Here's how the part is built. I have some questions about the finished solid (model axes, mm). A direction names the side the tool comes from. Coordinates: 2 decimals unless noted, no trailing zeros. Order: outer loops, then holes, each group sorted by start corner. A loop starts at its lowest first (then second) coordinate and runs counter-clockwise, first axis right, second up. Notation, with made-up numbers: (3.5, 5.25) - (31.5, 5.25) arc R25 ccw to (31.5, 17.25) - close; hole circle Ø3 at (-2.75, -19.75). An arc over 180 degrees is marked (long way). Answer as CSV lines item,"result". Start each with the question number.
Item 1: I need wall thicknesses on line 1 (X direction, y = 9, z = -2.25); line 2 (X direction, y = -3, z = 7); line 3 (X direction, y = 0.5, z = 13). Which ranges of each line are inside material? Lowest first, please.
Item 2: We'd pull the mould along X, two halves only. Please class faces 1 (the face through (-2.56, -1.03, 10.52)), 2 (the face through (0, 11, -10)), 3 (the face through (5.925, -0.944, 14.44)): pulls with the +X half, pulls with the -X half, needs draft (parallel to the pull), parting line crosses it, or undercut.
Item 3: On a 3-axis mill with a long thin cutter (end or side, diameter ignored), from which of +Z, -Z, +X, -X, +Y, -Y can I reach the whole of each face in a straight line? I mean faces 4 (the face through (5, 0, 0)), 5 (the face through (5.771, -0.712, 13.565)), 6 (the face through (3, -1, 16.6)), 7 (the face through (-5.78, -0.66, 15.33)), 8 (the face through (0, 8, 2.7)). Say none if no direction works.
Item 4: Imagine slicing it at D-D on y = 15. List the corners of the cut face in (x, z) for me.
Item 5: Imagine slicing it at C-C on y = 6. List the corners of the cut face in (x, z) for me.
Item 6: I'm going to push flat-ended pins straight in: pin 1 (3 mm diameter, centred on x = -6, y = 3, fed in from -Z); pin 2 (1 mm diameter, centred on y = -4.5, z = 9.5, fed in from -X); pin 3 (3.5 mm diameter, centred on y = 3.5, z = 10, fed in from +X); pin 4 (1.1 mm diameter, centred on x = 0, z = -0.5, fed in from -Y). Where does each tip first touch, or does it pass through?
from build123d import *

# Parameters (mm, degrees)
BOX_W             = 5.2
BOX_H             = 5
BOX_DEPTH         = 13
BOX003_W          = 2.1
BOX003_H          = 5
BOX003_DEPTH      = 13
CYLINDER003_R     = 2.76
CYLINDER003_DEPTH = 13.6
CYLINDER002_R     = 6
CYLINDER002_DEPTH = 2
CYLINDER001_R     = 7.4
CYLINDER001_DEPTH = 2.68
CYLINDER_R        = 5.6
CYLINDER_DEPTH    = 16.6
BOX002_W          = 3
BOX002_H          = 2
BOX002_DEPTH      = 4
BOX001_W          = 3
BOX001_H          = 29
BOX001_DEPTH      = 10
FILLET_1_R        = 9
FILLET_2_R        = 6
FILLET_3_R        = 2
FILLET001_R       = 2
FILLET002_R       = 2
FILLET003_R       = 1
CHAMFER_SIZE      = 0.3


with BuildPart() as box:
    # Box → Box (new body)
    with BuildSketch(Plane(origin=(-2.6, 1, 4.6), x_dir=(1, 0, 0), z_dir=(0, 0, 1))):
        with Locations((2.6, 2.5)):
            Rectangle(BOX_W, BOX_H)
    extrude(amount=BOX_DEPTH)


with BuildPart() as box003:
    # Box003 → Box003 (new body)
    with BuildSketch(Plane(origin=(-1.1, -7, 4.6), x_dir=(1, 0, 0), z_dir=(0, 0, 1))):
        with Locations((1.05, 2.5)):
            Rectangle(BOX003_W, BOX003_H)
    extrude(amount=BOX003_DEPTH)


with BuildPart() as fusion001:
    # Cylinder003 → Cylinder003 (new body)
    with BuildSketch(Plane.XY.offset(4.6)):
        Circle(CYLINDER003_R)
    extrude(amount=CYLINDER003_DEPTH)

    # Fusion001: union Box, Box003
    add(box.part)
    add(box003.part)


with BuildPart() as cylinder002:
    # Cylinder002 → Cylinder002 (new body)
    with BuildSketch(Plane.XY.offset(13.45)):
        Circle(CYLINDER002_R)
    extrude(amount=CYLINDER002_DEPTH)


with BuildPart() as base:
    # Cylinder001 → Cylinder001 (new body)
    with BuildSketch(Plane.XY):
        Circle(CYLINDER001_R)
    extrude(amount=CYLINDER001_DEPTH)


with BuildPart() as cut:
    # Cylinder → Cylinder (new body)
    with BuildSketch(Plane.XY):
        Circle(CYLINDER_R)
    extrude(amount=CYLINDER_DEPTH)

    # Fusion: union Cylinder002, base
    add(cylinder002.part)
    add(base.part)

    # Cut: cut Fusion001
    add(fusion001.part, mode=Mode.SUBTRACT)


with BuildPart() as obj1:
    # Box002 → Box002 (new body)
    with BuildSketch(Plane(origin=(-1.5, 7, -1.3), x_dir=(1, 0, 0), z_dir=(0, 0, 1))):
        with Locations((1.5, 1)):
            Rectangle(BOX002_W, BOX002_H)
    extrude(amount=BOX002_DEPTH)


with BuildPart() as chamfer_body:
    # Box001 → Box001 (new body)
    with BuildSketch(Plane(origin=(-1.5, -7.38, -10), x_dir=(1, 0, 0), z_dir=(0, 0, 1))):
        with Locations((1.5, 14.5)):
            Rectangle(BOX001_W, BOX001_H)
    extrude(amount=BOX001_DEPTH)

    # Fillet 1
    fillet_1_edges = [chamfer_body.edges().sort_by_distance(p)[0] for p in [
        (0, -7.38, -10),
    ]]
    fillet(fillet_1_edges, radius=FILLET_1_R)

    # Fillet 2
    fillet_2_edges = [chamfer_body.edges().sort_by_distance(p)[0] for p in [
        (0, 21.62, 0),
    ]]
    fillet(fillet_2_edges, radius=FILLET_2_R)

    # Fillet 3
    fillet_3_edges = [chamfer_body.edges().sort_by_distance(p)[0] for p in [
        (0, 21.62, -10),
    ]]
    fillet(fillet_3_edges, radius=FILLET_3_R)

    # Fusion002: union obj1
    add(obj1.part)

    # Fillet001
    fillet001_edges = [chamfer_body.edges().sort_by_distance(p)[0] for p in [
        (0, 9, 0),
    ]]
    fillet(fillet001_edges, radius=FILLET001_R)

    # Fusion003: union Cut
    add(cut.part)

    # Fillet002
    fillet002_edges = [chamfer_body.edges().sort_by_distance(p)[0] for p in [
        (1.5, 0, 0),
        (-1.5, 0, 0),
    ]]
    fillet(fillet002_edges, radius=FILLET002_R)

    # Fillet003
    fillet003_edges = [chamfer_body.edges().sort_by_distance(p)[0] for p in [
        (4.298837, -3.588872, 16.6),
        (4.791659, 2.898275, 16.6),
        (-5.543193, -0.795617, 16.6),
    ]]
    fillet(fillet003_edges, radius=FILLET003_R)

    # Chamfer
    chamfer_edges = [chamfer_body.edges().sort_by_distance(p)[0] for p in [
        (4.582576, -3.872983, 15.45),
        (4.582576, -3.872983, 13.45),
        (-5.947878, -0.789143, 13.45),
        (-5.947878, -0.789143, 15.45),
    ]]
    chamfer(chamfer_edges, length=CHAMFER_SIZE)


solid = chamfer_body.part
Responses:
1,line 1,"x = -1.5 to 1.5"
1,line 2,"x = -4.73 to -1.1, 1 to 4.73"
1,line 3,"x = -5.58 to -2.71, 2.71 to 5.58"
2,face 1,"undercut"
2,face 2,"needs draft"
2,face 3,"pulls with the +X half"
3,face 4,"-Z, +X, +Y, -Y"
3,face 5,"+X"
3,face 6,"+Z, +X, -X, +Y, -Y"
3,face 7,"+Z, -X"
3,face 8,"+Z, +X, -X, +Y"
4,outline,"(-1.5, -10) - (1.5, -10) - (1.5, 0) - (-1.5, 0) - close"
5,outline,"(-4.33, 0) - (-3.5, 0) arc R2 cw to (-1.5, -2) - (-1.5, -10) - (1.5, -10) - (1.5, -2) arc R2 cw to (3.5, 0) - (4.33, 0) - (4.33, 2.68) - (-4.33, 2.68) - close"
6,pin 1,"stops at z = 0"
6,pin 2,"stops at x = -3.92"
6,pin 3,"stops at x = 5.32"
6,pin 4,"stops at y = -7.4"
